```python
from build123d import *

# Parameters (mm, degrees)
F0_R     = 3
F1_DEPTH = 2
F2_W     = 4
F2_H     = 25
F3_DEPTH = 70
F5_DEPTH = 8
F6_R     = 12.49999
F7_R     = 2.5
F8_DEPTH = 4


# Not quite as in the source:
# - a fillet or chamfer is up to 0.001 mm smaller than in the source, because OpenCascade refuses the exact size
# - a feature names something its author has since deleted; it is built from what else it names


with BuildPart() as f1:
    # F0 (on Top) → F1 (new body)
    with BuildSketch(Plane.XY):
        with BuildLine():
            ThreePointArc((0, -12.5), (8.8388347648, -8.8388347648), (12.5, 0))
            ThreePointArc((12.5, 0), (8.8388347648, 8.8388347648), (0, 12.5))
            ThreePointArc((0, 12.5), (-12.5, 0), (0, -12.5))
        make_face()
        with BuildLine():
            ThreePointArc((1.4953181783, 9.3815789474), (7.2268777039, 6.1662175321), (9.5, 0))
            ThreePointArc((9.5, 0), (7.2268777039, -6.1662175321), (1.4953181783, -9.3815789474))
            ThreePointArc((1.4953181783, -9.3815789474), (1.4988290876, -9.4407432173), (1.5, -9.5))
            ThreePointArc((1.5, -9.5), (-0.0592567827, -10.9988290876), (-1.4953181783, -9.3815789474))
            ThreePointArc((-1.4953181783, -9.3815789474), (-7.2268777039, -6.1662175321), (-9.5, 0))
            ThreePointArc((-9.5, 0), (-7.2268777039, 6.1662175321), (-1.4953181783, 9.3815789474))
            ThreePointArc((-1.4953181783, 9.3815789474), (-0.0592567827, 10.9988290876), (1.5, 9.5))
            ThreePointArc((1.5, 9.5), (1.4988290876, 9.4407432173), (1.4953181783, 9.3815789474))
        make_face(mode=Mode.SUBTRACT)
        with BuildLine():
            ThreePointArc((0, 12.5), (8.8388347648, 8.8388347648), (12.5, 0))
            ThreePointArc((12.5, 0), (8.8388347648, -8.8388347648), (0, -12.5))
            Line((0, -12.5), (19, -12.5))
            Line((19, -12.5), (19, 12.5))
            Line((19, 12.5), (0, 12.5))
        make_face()
        with BuildLine():
            ThreePointArc((7.859375, -1.4933936552), (6.5, 0), (7.859375, 1.4933936552))
            ThreePointArc((7.859375, 1.4933936552), (5.1016100823, 6.1622702446), (1.34e-08, 8))
            ThreePointArc((1.34e-08, 8), (-5.101610072, 6.1622702532), (-7.859375, 1.4933936552))
            ThreePointArc((-7.859375, 1.4933936552), (-6.8907350407, 1.0097184013), (-6.5, 0))
            ThreePointArc((-6.5, 0), (-6.8907350407, -1.0097184013), (-7.859375, -1.4933936552))
            ThreePointArc((-7.859375, -1.4933936552), (-5.1016100771, -6.1622702489), (0, -8))
            ThreePointArc((0, -8), (5.1016100771, -6.1622702489), (7.859375, -1.4933936552))
        make_face()
        Circle(F0_R, mode=Mode.SUBTRACT)
        with BuildLine():
            ThreePointArc((7.859375, 1.4933936552), (9.0097184013, 1.1092649593), (9.5, 0))
            ThreePointArc((9.5, 0), (7.2268777039, 6.1662175321), (1.4953181783, 9.3815789474))
            ThreePointArc((1.4953181783, 9.3815789474), (1.0179313437, 8.3982669201), (1.34e-08, 8))
            ThreePointArc((1.34e-08, 8), (5.1016100823, 6.1622702446), (7.859375, 1.4933936552))
        make_face()
        with BuildLine():
            ThreePointArc((1.4953181783, -9.3815789474), (7.2268777039, -6.1662175321), (9.5, 0))
            ThreePointArc((9.5, 0), (9.0097184013, -1.1092649593), (7.859375, -1.4933936552))
            ThreePointArc((7.859375, -1.4933936552), (5.1016100771, -6.1622702489), (0, -8))
            ThreePointArc((0, -8), (1.0179313388, -8.3982669155), (1.4953181783, -9.3815789474))
        make_face()
        with BuildLine():
            ThreePointArc((1.34e-08, 8), (-1.0179313339, 8.3982669109), (-1.4953181783, 9.3815789474))
            ThreePointArc((-1.4953181783, 9.3815789474), (-7.2268777039, 6.1662175321), (-9.5, 0))
            ThreePointArc((-9.5, 0), (-9.0097184013, 1.1092649593), (-7.859375, 1.4933936552))
            ThreePointArc((-7.859375, 1.4933936552), (-5.101610072, 6.1622702532), (1.34e-08, 8))
        make_face()
        with BuildLine():
            ThreePointArc((-9.5, 0), (-7.2268777039, -6.1662175321), (-1.4953181783, -9.3815789474))
            ThreePointArc((-1.4953181783, -9.3815789474), (-1.0179313388, -8.3982669155), (0, -8))
            ThreePointArc((0, -8), (-5.1016100771, -6.1622702489), (-7.859375, -1.4933936552))
            ThreePointArc((-7.859375, -1.4933936552), (-9.0097184013, -1.1092649593), (-9.5, 0))
        make_face()
    extrude(amount=F1_DEPTH)

    # F2 (on face) → F3 (join)
    with BuildSketch(Plane.XY.offset(2)):
        with Locations((17, 0)):
            Rectangle(F2_W, F2_H)
    extrude(amount=F3_DEPTH)

    # F4 (on face) → F5 (join)
    with BuildSketch(Plane(origin=(15, 0, 0), x_dir=(0, -1, 0), z_dir=(-1, 0, 0))):
        with BuildLine():
            Line((-2.5, 59.5), (2.5, 59.5))
            ThreePointArc((2.5, 59.5), (0, 62), (-2.5, 59.5))
        make_face()
    extrude(amount=F5_DEPTH)

    # F6 (radius 12.5 in the source; OpenCascade refuses exactly that, so slightly less here)
    f6_edges = [f1.edges().sort_by_distance(p)[0] for p in [
        (17, -12.5, 72),
        (17, 12.5, 72),
    ]]
    fillet(f6_edges, radius=F6_R)

    # F7 (on face) → F8 (cut, through all)
    with BuildSketch(Plane.YZ.offset(19)):
        with Locations((0, 44)):
            Circle(F7_R)
    extrude(amount=-F8_DEPTH, mode=Mode.SUBTRACT)


solid = f1.part
```
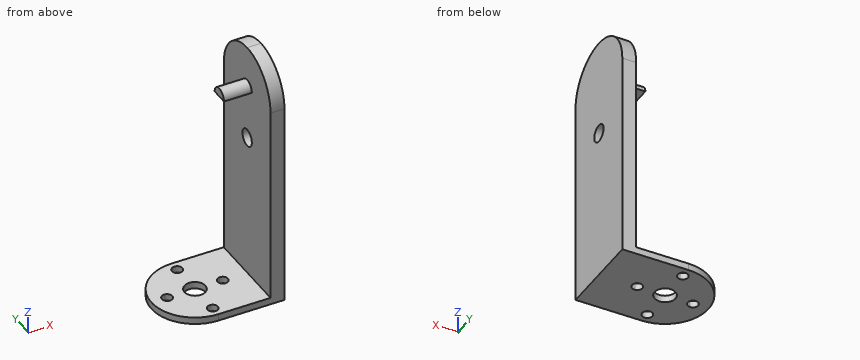
Part model, mm, in its own coordinate system. Coordinates: 2 decimals unless noted, no trailing zeros. Write each loop counter-clockwise with the first axis right and the second up, starting at its lowest first coordinate (ties: lowest second). Pieces come first, ordered by that corner, then holes.
Item 1: Probe line 1 (Z direction, x = 17.7, y = 0); line 2 (Z direction, x = 2.5, y = -5.5); line 3 (X direction, y = -1.5, z = 56.5). List the from-to ranges inside material, lowest first.
Item 2: Pin check, flat tips, straight feed: pin 1 (6 mm diameter, centred on x = -1, y = -7.5, fed in from +Z); pin 2 (2 mm diameter, centred on y = -1, z = 60.5, fed in from -X); pin 3 (7.5 mm diameter, centred on y = -2, z = 34.5, fed in from -X). Stop position of each tip, or through.
Item 3: Slice it at D-D (x = 4.5). Write the cut outline in (y, z).
Item 4: Slice it at B-B (y = -5.25). Write the cut outline in (x, z), and give its area (3 significant figures).
Item 5: Slice it at A-A (z = 44). Write the cut outline in (x, y), and give its area (3 significant figures).
Item 6: Slice it at C-C (z = 32). Write the cut outline in (x, y).
Results found:
1. line 1: z = 0 to 41.5, 46.5 to 72
1. line 2: z = 0 to 2
1. line 3: x = 15 to 19
2. pin 1: stops at z = 2
2. pin 2: stops at x = 7
2. pin 3: stops at x = 15
3. outline: (-12.5, 0) - (12.5, 0) - (12.5, 2) - (-12.5, 2) - close
4. outline: (-11.34, 0) - (19, 0) - (19, 70.84) - (15, 70.84) - (15, 2) - (-11.34, 2) - close
4. area: 336 mm2
5. outline: (15, -12.5) - (19, -12.5) - (19, -2.5) - (15, -2.5) - close; (15, 2.5) - (19, 2.5) - (19, 12.5) - (15, 12.5) - close
5. area: 80.0 mm2
6. outline: (15, -12.5) - (19, -12.5) - (19, 12.5) - (15, 12.5) - close
